```python
from build123d import *

# Parameters (mm, degrees)
SKETCH1_R                      = 2.75
SKETCH1_R_2                    = 5.1
BOSS_EXTRUDE1_DEPTH            = 8
CBORE_FOR_M2_SHCS1_D           = 2.4
CBORE_FOR_M2_SHCS1_CBORE_D     = 4.4
CBORE_FOR_M2_SHCS1_CBORE_DEPTH = 2
CHAMFER1_SIZE                  = 1


with BuildPart() as part:
    # Sketch1 → Boss-Extrude1 (new body)
    with BuildSketch(Plane.XY):
        with BuildLine():
            Line((9.9380799, -1.111111111), (14.90711985, 43.333333333))
            ThreePointArc((14.90711985, 43.333333333), (0, 60), (-14.90711985, 43.333333333))
            Line((-14.90711985, 43.333333333), (-9.9380799, -1.111111111))
            ThreePointArc((-9.9380799, -1.111111111), (0, -10), (9.9380799, -1.111111111))
        make_face()
        Circle(SKETCH1_R, mode=Mode.SUBTRACT)
        with Locations((0, 45)):
            Circle(SKETCH1_R_2, mode=Mode.SUBTRACT)
    extrude(amount=BOSS_EXTRUDE1_DEPTH)

    # CBORE for M2 SHCS1 (through all)
    with Locations(Plane.XY.offset(8)):
        with Locations((0, -6), (-6, 0), (0, 6), (6, 0)):
            CounterBoreHole(CBORE_FOR_M2_SHCS1_D / 2, CBORE_FOR_M2_SHCS1_CBORE_D / 2, CBORE_FOR_M2_SHCS1_CBORE_DEPTH)

    # Chamfer1
    chamfer1_edges = [part.edges().sort_by_distance(p)[0] for p in [
        (12.422599875, 21.111111111, 8),
        (0, 60, 8),
        (-12.422599875, 21.111111111, 8),
        (0, -10, 8),
        (0, -10, 0),
        (-12.422599875, 21.111111111, 0),
        (0, 60, 0),
        (12.422599875, 21.111111111, 0),
    ]]
    chamfer(chamfer1_edges, length=CHAMFER1_SIZE)


solid = part.part
```
The listing builds one solid part. Answer for the finished solid, in the listing's coordinates (mm). A direction names the side the tool comes from. Round coordinates to 2 decimals unless told otherwise and drop trailing zeros. Write each loop counter-clockwise with the first axis right and the second up, starting at its lowest first coordinate (ties: lowest second). Pieces come first, ordered by that corner, then holes. Notation, with made-up numbers: (20, 61) -> (40, 61) arc R15 ccw to (40, 73) -> close; hole circle Ø6 at (37.5, -35.5). An arc over 180 degrees is marked (long way). Answer as a JSON object with one key per item and string values. Group by question number.
Q1. Each of these flat-tipped pins is pushed along its axis until it touches: pin 1 Ø1 at (x, z) = (6, 4.5) entering from +Y; pin 2 Ø3 at (x, y) = (6, 0) entering from +Z; pin 3 Ø1 at (y, z) = (51, 6.5) entering from +X. Where does it stop, or does it pass through?
Q2. Section A-A (y = 45) is taken. Write down the section's boundary in (x, z).
Q3. Straight lines are drawn through the part: line 1 along Y through (x, z) = (2, 4); line 2 along Y through (x, z) = (-7, 7); line 3 along Y through (x, z) = (-0.5, 6.5). For each, find the intervals that lie inside material, in ascending order.
Q4. Section D-D (y = 6) is taken. Write down the section's boundary in (x, z).
Q5. Which of the six approach directions +Z, -Z, +X, -X, +Y, -Y give full straight-line access (tool end or side, diameter ignored) to faces 1 (the face through (1.183, 7.855, 7.014)), 2 (the face through (-1, 50, 4))?
Q6. Determine the mould class of faces 3 (the face through (-0.477, -8.148, 7.014)), 4 (the face through (11.88, 20.86, 7.51)), 5 (the face through (1, -7, 6)), 6 (the face through (0, 25, 0)) for opening direction Y: pulls with the +Y half, pulls with the -Y half, needs draft (parallel to the pull), parting line crosses it, or undercut.
Q7. Section C-C (y = 33) is taken. Write down the section's boundary in (x, z), plus the area to 3 significant figures.
Q8. Section B-B (x = 0) is taken. Count the separate pieces of the cut face and the enclosed holes in it, plus the area to 3 significant figures.
Check values:
{
 "1": {"pin 1": "y = 58.96", "pin 2": "z = 6", "pin 3": "x = 13.96"},
 "2": {"outline": "(-15, 1) -> (-14, 0) -> (-5.1, 0) -> (-5.1, 8) -> (-14, 8) -> (-15, 7) -> close; (5.1, 0) -> (14, 0) -> (15, 1) -> (15, 7) -> (14, 8) -> (5.1, 8) -> close"},
 "3": {"line 1": "-9.8 to -1.89, 1.89 to 40.31, 49.69 to 59.87", "line 2": "-7.14 to -1.96, 1.96 to 58.27", "line 3": "-9.99 to -8.14, -3.86 to -2.7, 2.7 to 3.86, 8.14 to 39.92, 50.08 to 59.99"},
 "4": {"outline": "(-10.73, 1) -> (-9.73, 0) -> (-1.2, 0) -> (-1.2, 6) -> (-2.2, 6) -> (-2.2, 8) -> (-9.73, 8) -> (-10.73, 7) -> close; (1.2, 0) -> (9.73, 0) -> (10.73, 1) -> (10.73, 7) -> (9.73, 8) -> (2.2, 8) -> (2.2, 6) -> (1.2, 6) -> close"},
 "5": {"face 1": "+Z", "face 2": "+Z, -Z"},
 "6": {"face 3": "undercut", "face 4": "pulls with the -Y half", "face 5": "undercut", "face 6": "needs draft"},
 "7": {"outline": "(-13.75, 1) -> (-12.75, 0) -> (12.75, 0) -> (13.75, 1) -> (13.75, 7) -> (12.75, 8) -> (-12.75, 8) -> (-13.75, 7) -> close", "area": "218 mm^2"},
 "8": {"separate pieces": "5", "enclosed holes": "0", "area": "386 mm^2"}
}
